Input: dimensioned drawing with shaded views. Units: mm. Origin: part minimum x, y, z. A direction names the side the tool comes from. Round coordinates to 2 decimals unless told otherwise and drop trailing zeros. Loops run counter-clockwise (first coordinate to the right, second up) from the corner with the lowest first, then second, coordinate; pieces in that order, holes last. Notation, with made-up numbers: M 11.25,34 L 54.25,34 A16 cw 54.25,46 Z; hole C 68,5.25 d11. An arc over 180 degrees is marked long. Answer as a JSON object with one key per item and string values.
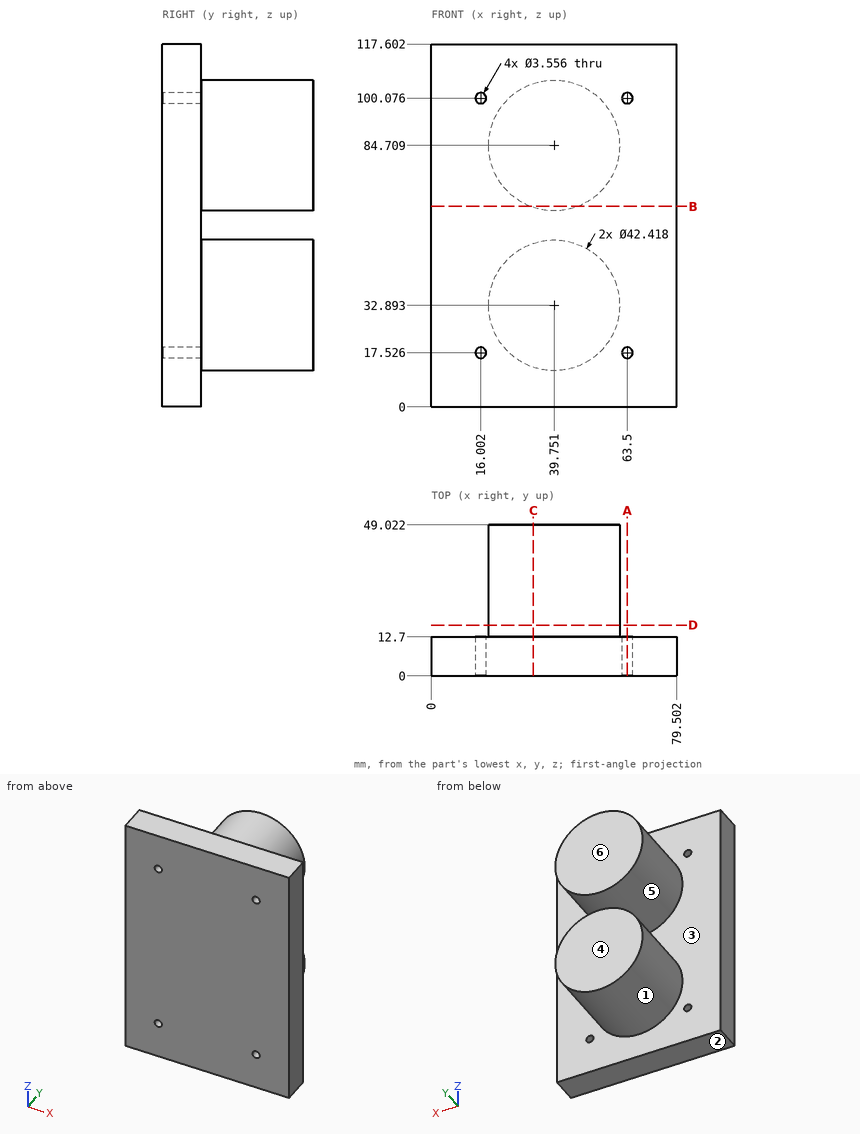
Item 1: Section D-D on y = 16.5. Return the cut outline in (x, z).
Answer sheet:
{"outline": "C 39.75,32.89 d42.42; C 39.75,84.71 d42.42"}
Item 2: Contact query for flat-ended pins moving along their axis: pin 1 Ø2 at (x, y) = (28.5, 21) entering from -Z; pin 2 Ø4.5 at (x, z) = (16.002, 100.076) entering from +Y; pin 3 Ø2 at (x, z) = (63.5, 17.526) entering from -Y; pin 4 Ø4 at (x, y) = (47.5, 36) entering from +Z. Output: stop coordinate, or through.
Answer sheet:
{"pin 1": "stops at z = 14.33", "pin 2": "stops at y = 12.7", "pin 3": "passes through", "pin 4": "stops at z = 105.12"}
Item 3: Line query: probe 1 along Z at (x, y) = (63, 6); probe 2 along X at (y, z) = (35, 33); probe 3 along Y at (x, z) = (61, 17). Output: solid intervals per line, ascending. Write a range as from..to.
Answer sheet:
{"probe 1": "z = 0..15.82, 19.23..98.37, 101.78..117.6", "probe 2": "x = 18.54..60.96", "probe 3": "y = 0..12.7"}
Item 4: Section C-C on x = 33. Return the cut outline in (y, z).
Answer sheet:
{"outline": "M 0,0 L 12.7,0 L 12.7,12.79 L 49.02,12.79 L 49.02,53 L 12.7,53 L 12.7,64.6 L 49.02,64.6 L 49.02,104.81 L 12.7,104.81 L 12.7,117.6 L 0,117.6 Z"}
Item 5: Section A-A on x = 63.5. Return the cut outline in (y, z).
Answer sheet:
{"outline": "M 0,0 L 12.7,0 L 12.7,15.75 L 0,15.75 Z; M 0,19.3 L 12.7,19.3 L 12.7,98.3 L 0,98.3 Z; M 0,101.85 L 12.7,101.85 L 12.7,117.6 L 0,117.6 Z"}
Item 6: Section B-B on z = 65. Return the cut outline in (x, y), then the cut area to 3 significant figures.
Answer sheet:
{"outline": "M 0,0 L 79.5,0 L 79.5,12.7 L 47.59,12.7 L 47.59,49.02 L 31.92,49.02 L 31.92,12.7 L 0,12.7 Z", "area": "1,580 mm²"}
Item 7: Pull-direction query (Z, two-part tool) for the marked faces 1, 2, 3 and 4; classes: pulls with the +Z half, pulls with the -Z half, needs draft (parallel to the pull), parting line crosses it, or undercut.
Answer sheet:
{"face 1": "undercut", "face 2": "pulls with the -Z half", "face 3": "undercut", "face 4": "needs draft"}
Item 8: Access query for the marked faces 5 and 6. Directions: +Z, -Z, +X, -X, +Y, -Y. A direction counts if a zero-diameter tool reaches every point of the face in a straight line with its end or side. Return the directions, or none.
Answer sheet:
{"face 5": "+Y", "face 6": "+Z, -Z, +X, -X, +Y"}
